Autodesk Inventor part; units mm, degrees
ref_plane "YZ Plane" through (0, 0, 0) normal (1, 0, 0) x (0, 1, 0)
ref_plane "XZ Plane" through (0, 0, 0) normal (0, 1, 0) x (-1, 0, 0)
ref_plane "XY Plane" through (0, 0, 0) normal (0, 0, 1) x (1, 0, 0)
sketch "Szkic1" plane through (0, 0, 0) normal (0, 1, 0) x (-1, 0, 0)
  circle A0 centre (0, 0) radius 18.5
  circle A1 centre (0, 0) radius 15.125
  line L0 (15.125, 0) -> (7.5625, -13.0986)
  line L1 (7.5625, -13.0986) -> (-7.5625, -13.0986)
  line L2 (-7.5625, -13.0986) -> (-15.125, 0)
  line L3 (-15.125, 0) -> (-7.5625, 13.0986)
  line L4 (-7.5625, 13.0986) -> (7.5625, 13.0986)
  line L5 (7.5625, 13.0986) -> (15.125, 0)
  circle A2 centre (-15.125, 0) radius 1.75
  circle A3 centre (-7.5625, -13.0986) radius 1.75
  circle A4 centre (7.5625, -13.0986) radius 1.75
  line L6 (-18.5, 0) -> (-29.5, 0)
  line L7 (-29.5, 0) -> (-29.5, -18.5)
  line L8 (-29.5, -18.5) -> (-18.5, -18.5)
  line L9 (-18.5, -18.5) -> (-18.5, 0)
  line L10 (-29.5, -18.5) -> (-26, -18.5)
  line L11 (-26, -18.5) -> (-26, 0)
  line L12 (-26, 0) -> (-29.5, 0)
  line L13 (-29.5, 0) -> (-29.5, -18.5)
  line L14 (-26, -18.5) -> (-22, -18.5)
  line L15 (-22, -18.5) -> (-22, 0)
  line L16 (-22, 0) -> (-26, 0)
  line L17 (-26, 0) -> (-26, -18.5)
  line L18 (-18.5, 0) -> (-29.5, 0)
  line L19 (-29.5, 0) -> (-29.5, 15)
  line L20 (7.5625, -13.0986) -> (-18.5, -13.0986)
  line L21 (-18.5, -13.0986) -> (-18.5, -16.0986)
  line L22 (-18.5, -16.0986) -> (7.5625, -16.0986)
  line L23 (7.5625, -16.0986) -> (7.5625, -13.0986)
  line L24 (7.5625, -10.0986) -> (7.5625, -16.0986)
  line L25 (7.5625, -10.0986) -> (-18.5, -10.0986)
  line L26 (-18.5, -10.0986) -> (-18.5, -13.0986)
  line L27 (-18.5, -13.0986) -> (7.5625, -13.0986)
  line L28 (7.5625, -13.0986) -> (7.5625, -10.0986)
  line L29 (7.5625, -10.0986) -> (10.5625, -10.0986)
  line L30 (10.5625, -10.0986) -> (10.5625, -16.0986)
  line L31 (10.5625, -16.0986) -> (7.5625, -16.0986)
  line L32 (7.5625, -16.0986) -> (7.5625, -10.0986)
  line L33 (10.5625, -10.0986) -> (-18.5, 6.6806)
  line L34 (-18.5, -18.5) -> (10.5625, -16.0986)
  line L35 (-18.5, 6.6806) -> (-29.5, 13.0315)
  line L36 (-29.5, 0) -> (-18.5, 0)
  line L37 (-18.5, 0) -> (-18.5, 6.6806)
  line L38 (-18.5, 6.6806) -> (-29.5, 6.6806)
  line L39 (-29.5, 6.6806) -> (-29.5, 0)
  point P0 (-9.3125, -13.0986)
  point P1 (-5.8125, -13.0986)
  point P2 (5.8125, -13.0986)
  point P3 (7.5625, -14.8486)
  dimension "d0" = 37
  dimension "d1" = 30.25
  dimension "d2" = 3.5
  dimension "d3" = 3.5
  dimension "d4" = 3.5
  dimension "d5" = 11
  dimension "d6" = 3.5
  dimension "d7" = 4
  dimension "d9" = 3
  dimension "d10" = 3
  dimension "d12" = 3
  dimension "d13" = 30
extrude "Wyciągnięcie proste1" add sketch "Szkic1" along normal blind 3.5 contours L33 A1 A2 L25 A0 | A0 L37 L33 | L30 L31 A0 | A0 L31 L23 A4 A1 L30 | L9 L8 L15 L6 | A0 L25 L9 | L6 L19 L38 L37 | L33 L3 A2 A1 | L31 L34 A0 | A0 L34 L22 L31 | A1 A4 L0 L29 L30 | L25 A1 A3 L20 A0 | A0 L20 L9 L25 | L15 L8 L11 L6 | L33 L0 L29 L25 L2 A2 L3 | L22 A0 L20 A3 A1 A4 L23 | L29 L0 L33 | A0 L22 L9 L20 | L25 L2 A3 A1 | A1 A2 L2 L25 | L11 L8 L7 L6 | L34 L9 L22 A0 | A4 L24 L29 L0 | L25 L24 A4 L1 A3 L2 | A1 A3 L1 A4
sketch "Szkic2" plane through (0, 3.5, 0) normal (0, 1, 0) x (1, 0, 0)
  line L0 (18.5, -6.6806) -> (29.5, -6.6806)
  line L1 (18.5, 18.5) -> (-10.5625, 16.0986)
  line L2 (29.5, -6.6806) -> (18.5, -6.6806)
  line L3 (18.5, -6.6806) -> (18.5, 18.5)
  line L4 (18.5, 18.5) -> (29.5, 18.5)
  line L5 (29.5, 18.5) -> (29.5, -6.6806)
  point P0 (0, 0)
extrude "Wyciągnięcie proste2" add sketch "Szkic2" along normal blind 74
sketch "Szkic3" plane through (0, 77.5, 0) normal (0, 1, 0) x (1, 0, 0)
  line L0 (18.5, -6.6806) -> (29.5, -6.6806)
  line L1 (29.5, 18.5) -> (18.5, 18.5)
  line L2 (26, -6.6806) -> (22, -6.6806)
  line L3 (22, -6.6806) -> (22, 18.5)
  line L4 (22, 18.5) -> (26, 18.5)
  line L5 (26, 18.5) -> (26, -6.6806)
  line L6 (18.5, 18.5) -> (18.5, -6.6806)
  point P0 (0, 0)
  dimension "d21" = 4
  dimension "d22" = 3.5
extrude "Wyciągnięcie proste3" cut sketch "Szkic3" against normal blind 60 contours L3 L1 L5 L0
sketch "Szkic4" plane through (0, 17.5, 0) normal (0, 1, 0) x (1, 0, 0)
  line L0 (26, 18.5) -> (26, -6.6806)
  line L1 (22, -6.6806) -> (22, 18.5)
  line L2 (22, 0) -> (22, 11.8194)
  line L3 (26, 11.8194) -> (26, 0)
  line L4 (26, -6.6806) -> (22, -6.6806)
  line L5 (22, 18.5) -> (26, 18.5)
  line L6 (22, 14.5) -> (26, 14.5)
  line L7 (26, 14.5) -> (26, -2.6806)
  line L8 (26, -2.6806) -> (22, -2.6806)
  line L9 (22, -2.6806) -> (22, 14.5)
  point P0 (0, 0)
  dimension "d29" = 4
  dimension "d30" = 4
extrude "Wyciągnięcie proste4" cut sketch "Szkic4" against normal blind 60 contours L0 L8 L1 L6
sketch "Szkic8" plane through (29.5, 0, 6.6806) normal (1, 0, 0) x (0, 0, -1)
  line L0 (-17, 23.5) -> (25.1806, 23.5)
  line L1 (25.1806, 0) -> (25.1806, 77.5)
  line L2 (6.6806, 0) -> (6.6806, 23.5)
  line L3 (6.6806, 18.5) -> (30.6806, 18.5)
  line L4 (30.6806, 18.5) -> (30.6806, 28.5)
  line L5 (30.6806, 28.5) -> (6.6806, 28.5)
  line L6 (6.6806, 28.5) -> (6.6806, 18.5)
  line L7 (6.6806, 18.5) -> (-17.3194, 18.5)
  line L8 (-17.3194, 18.5) -> (-17.3194, 28.5)
  line L9 (-17.3194, 28.5) -> (6.6806, 28.5)
  line L10 (6.6806, 28.5) -> (6.6806, 18.5)
  line L11 (30.6806, 23.5) -> (-17.3194, 23.5)
  line L12 (30.6806, 19.5) -> (-17.3194, 19.5)
  line L13 (-17.3194, 19.5) -> (-17.3194, 27.5)
  line L14 (-17.3194, 27.5) -> (30.6806, 27.5)
  line L15 (30.6806, 27.5) -> (30.6806, 19.5)
  point P0 (25.1806, 28.5)
  point P1 (25.1806, 18.5)
  point P2 (25.1806, 27.5)
  point P3 (25.1806, 19.5)
  point P4 (6.6806, 27.5)
  point P5 (6.6806, 19.5)
  dimension "d39" = 24
  dimension "d40" = 24
  dimension "d47" = 1
  dimension "d48" = 1
extrude "Wyciągnięcie proste6" add sketch "Szkic8" against normal blind 3.5 contours L11 L8 L14 L6 L0 | L0 L2 L12 L8 L11 | L11 L4 L12 L1 | L1 L14 L4 L11
sketch "Szkic9" plane through (26, 77.5, -18.5) normal (-1, 0, 0) x (0, 0, 1)
  line L0 (42.5, -58) -> (42.5, -50)
  line L1 (42.5, -54) -> (38.5, -54)
  circle A0 centre (38.5, -54) radius 2
  line L2 (-5.5, -50) -> (-5.5, -58)
  line L3 (-5.5, -54) -> (-1.5, -54)
  circle A1 centre (-1.5, -54) radius 2
  point P0 (18.5, -77.5)
  point P1 (42.5, -59)
  point P2 (42.5, -49)
  point P3 (-5.5, -49)
  point P4 (-5.5, -59)
  dimension "d43" = 4
  dimension "d44" = 4
  dimension "d45" = 4
  dimension "d46" = 4
extrude "Wyciągnięcie proste7" cut sketch "Szkic9" along normal mid plane 50
fillet "Zaokrąglenie3" radius 2 11 edges at (-10.5625, 1.75, -16.0986) (-10.5625, 1.75, -10.0986) (29.5, 0, -5.9097) (27.75, 19.5, 24) (27.75, 27.5, 24) (27.75, 19.5, -24) (27.75, 27.5, -24) (27.75, 77.5, -18.5) (27.75, 77.5, 6.6806) (20.25, 77.5, 6.6806) (20.25, 77.5, -18.5)
sketch "Szkic10" plane through (18.5, 3.5, -18.5) normal (-1, 0, 0) x (0, 0, 1)
  circle A0 centre (-1.5, 20) radius 2
  circle A1 centre (-1.5, 20) radius 3
  point P0 (18.5, -3.5)
  dimension "d52" = 6
extrude "Wyciągnięcie proste8" cut sketch "Szkic10" against normal blind 4 contours A0 | A1
sketch "Szkic11" plane through (29.5, 21.5, 24) normal (1, 0, 0) x (0, 0, -1)
  circle A0 centre (44, 2) radius 2
  line L0 (4.0189, 2) -> (44, 2)
  point P0 (24, -21.5)
  dimension "d55" = 39.9811
properties part number "nasilnikprzod1_new"
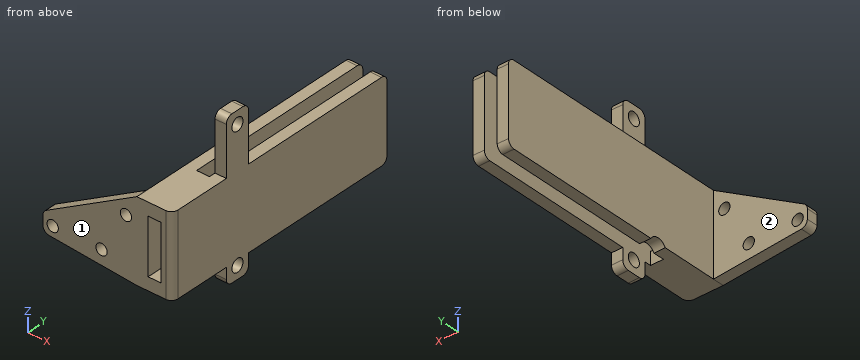
Source: CAD feature listing. Evaluate the final solid. Frame: model axes, mm. Face numbers are marked on the shaded views. A direction names the side the tool comes from. Give positions to 0.01 mm unless a question says otherwise; leave off trailing zeros. Order: outer loops, then holes, each group sorted by start corner. A loop starts at its lowest first (then second) coordinate and runs counter-clockwise, first axis right, second up.
(1) Material intervals for line 1 along Y through (x, z) = (27, 20); line 2 along X through (y, z) = (38.5, -15.5); line 3 along Z through (x, y) = (27, 46.5), sorted ascending.
(2) Access query for the marked faces 1 and 2. Directions: +Z, -Z, +X, -X, +Y, -Y. A direction counts if a zero-diameter tool reaches every point of the face in a straight line with its end or side. Return the directions, or none.
(3) Section query C-C (y = 6.5). Return the cut outline in (x, z), plus the area to 3 significant figures.
(4) Contact query for flat-ended pins moving along their axis: P1, Ø20, axis at y = 39, z = -4.5, coming from the -X side; P2, Ø1, axis at x = 23.5, z = -6, coming from the -Y side; P3, Ø2, axis at x = 23, y = 7, coming from the +Z side; P4, Ø1.2, axis at x = 23, z = -16, coming from the +Y side. Output: stop coordinate, or through.
(5) Section query A-A (y = 23.5). Return the cut outline in (x, z).
(6) Section query B-B (z = 20). Return the cut outline in (x, y), plus the area to 3 significant figures.
(7) Section query D-D (x = -3.5). Return the cut outline in (y, z).
Outcome:
1. line 1: y = 19.5 to 21.5, 25.5 to 27.5
1. line 2: x = 18.5 to 22, 26 to 29.5
1. line 3: z = -18.5 to 6.68
2. face 1: +Z, -Z, +X, -X, -Y
2. face 2: +Z, -Z, -X, +Y
3. outline: (18.5, -18.5) - (29.5, -18.5) - (29.5, 6.68) - (18.5, 6.68) - close; hole (22, -14.5) - (26, -14.5) - (26, 2.68) - (22, 2.68) - close
3. area: 208 mm2
4. P1: stops at x = 18.5
4. P2: passes through
4. P3: stops at z = 6.68
4. P4: stops at y = 17.5
5. outline: (18.5, -17) - (22, -17) - (22, 6.68) - (18.5, 6.68) - close; (26, -24) - (29.5, -24) - (29.5, -22) - (26, -22) - close; (26, -18) - (29.5, -18) - (29.5, 18) - (26, 18) - close; (26, 22) - (29.5, 22) - (29.5, 24) - (26, 24) - close
6. outline: (26, 19.5) - (29.5, 19.5) - (29.5, 21.5) - (26, 21.5) - close; (26, 25.5) - (29.5, 25.5) - (29.5, 27.5) - (26, 27.5) - close
6. area: 14.0 mm2
7. outline: (0, -16.68) - (3.5, -16.68) - (3.5, -6.02) - (0, -6.02) - close
